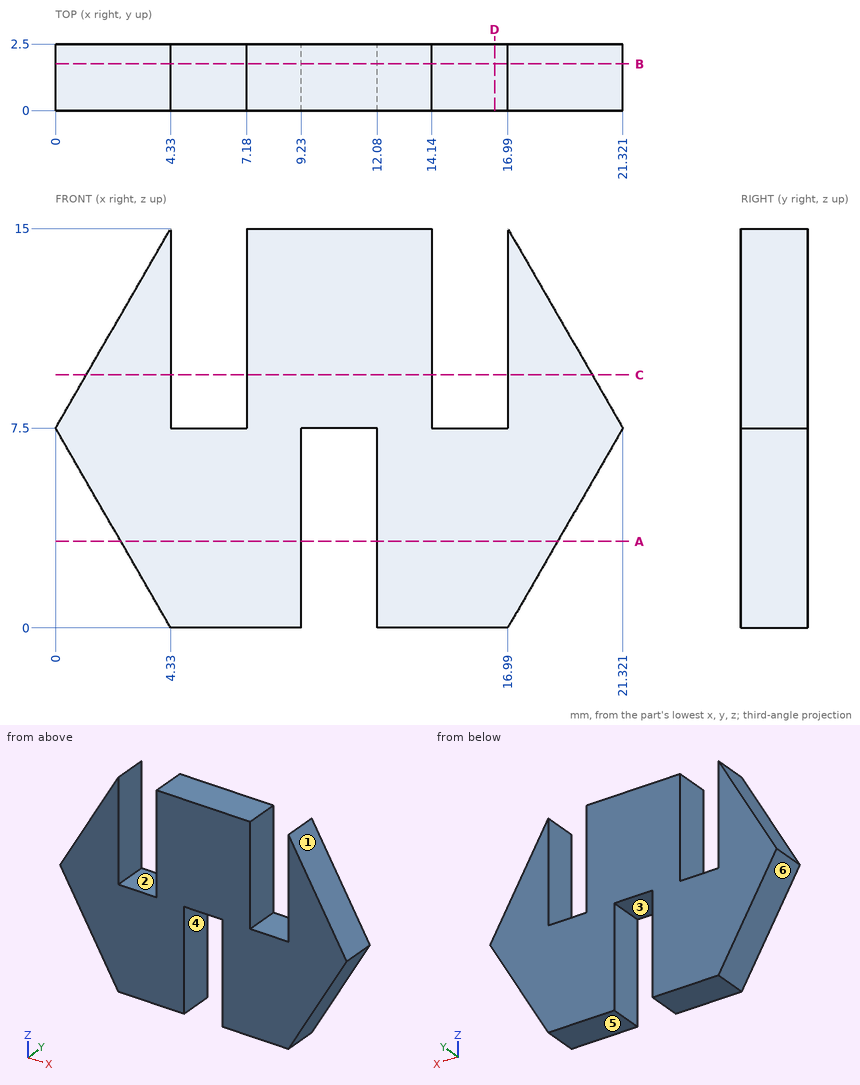
Here's the drawing with two shaded views (mm, measured from the low corner). I have some questions. A direction names the side the tool comes from. Give positions to 0.01 mm unless a question says otherwise; leave off trailing zeros. Order: outer loops, then holes, each group sorted by start corner. A loop starts at its lowest first (then second) coordinate and runs counter-clockwise, first axis right, second up. Notation, with made-up numbers: (-25.75, 55) - (30.25, 55) arc R25 ccw to (30.25, 90) - close; hole circle Ø6 at (-4, -18.75). An arc over 180 degrees is marked (long way). Use a Markdown table: item, result. Add a question column.
Q1. On a 3-axis mill with a long thin cutter (end or side, diameter ignored), from which of +Z, -Z, +X, -X, +Y, -Y can I reach the whole of each face in a straight line? I mean the marked faces 1, 2 and 3. Say none if no direction works.
Q2. If we section it at B-B on y = 1.75: Write out the boundary of the cut face in (x, z), plus the area to 3 significant figures.
Q3. Please list where these lines run through material, in increasing order: line 1 along X through (y, z) = (0.85, 13.75); line 2 along X through (y, z) = (1.55, 10.5); line 3 along Z through (x, y) = (11.75, 1.6).
Q4. If we section it at D-D on x = 16.5: Write out the boundary of the cut face in (y, z).
Q5. If we section it at A-A on z = 3.25: Write out the boundary of the cut face in (x, y), plus the area to 3 significant figures.
Q6. If we section it at C-C on z = 9.5: Write out the boundary of the cut face in (x, y) (1 decimal).
Q7. I'm going to push flat-ended pins straight in: pin 1 (1 mm diameter, centred on y = 1.5, z = 11.5, fed in from -X); pin 2 (1.2 mm diameter, centred on y = 1, z = 11, fed in from +X) (1 decimal); pin 3 (0.8 mm diameter, centred on x = 5, y = 0.5, fed in from +Z). Where does each tip first touch, or does it pass through?
Q8. If we mould it in two halves opening along X, with no side actions, what happens to the marked faces 4, 5 and 6? For each: released by +X, released by -X, zero draft, split by the parting line, or undercut.
Answers follow:
| question | item | result |
|---|---|---|
| 1 | face 1 | +Z, +X, +Y, -Y |
| 1 | face 2 | +Z, +Y, -Y |
| 1 | face 3 | -Z, +Y, -Y |
| 2 | outline | (0, 7.5) - (4.33, 0) - (9.23, 0) - (9.23, 7.5) - (12.08, 7.5) - (12.08, 0) - (16.99, 0) - (21.32, 7.5) - (16.99, 15) - (16.99, 7.5) - (14.14, 7.5) - (14.14, 15) - (7.18, 15) - (7.18, 7.5) - (4.33, 7.5) - (4.33, 15) - close |
| 2 | area | 191 mm^2 |
| 3 | line 1 | x = 3.61 to 4.33, 7.18 to 14.14, 16.99 to 17.71 |
| 3 | line 2 | x = 1.73 to 4.33, 7.18 to 14.14, 16.99 to 19.59 |
| 3 | line 3 | z = 7.5 to 15 |
| 4 | outline | (0, 0) - (2.5, 0) - (2.5, 7.5) - (0, 7.5) - close |
| 5 | outline | (2.45, 0) - (9.23, 0) - (9.23, 2.5) - (2.45, 2.5) - close; (12.08, 0) - (18.87, 0) - (18.87, 2.5) - (12.08, 2.5) - close |
| 5 | area | 33.9 mm^2 |
| 6 | outline | (1.2, 0) - (4.3, 0) - (4.3, 2.5) - (1.2, 2.5) - close; (7.2, 0) - (14.1, 0) - (14.1, 2.5) - (7.2, 2.5) - close; (17, 0) - (20.2, 0) - (20.2, 2.5) - (17, 2.5) - close |
| 7 | pin 1 | stops at x = 2.02 |
| 7 | pin 2 | stops at x = 19.6 |
| 7 | pin 3 | stops at z = 7.5 |
| 8 | face 4 | undercut |
| 8 | face 5 | zero draft |
| 8 | face 6 | released by -X |
